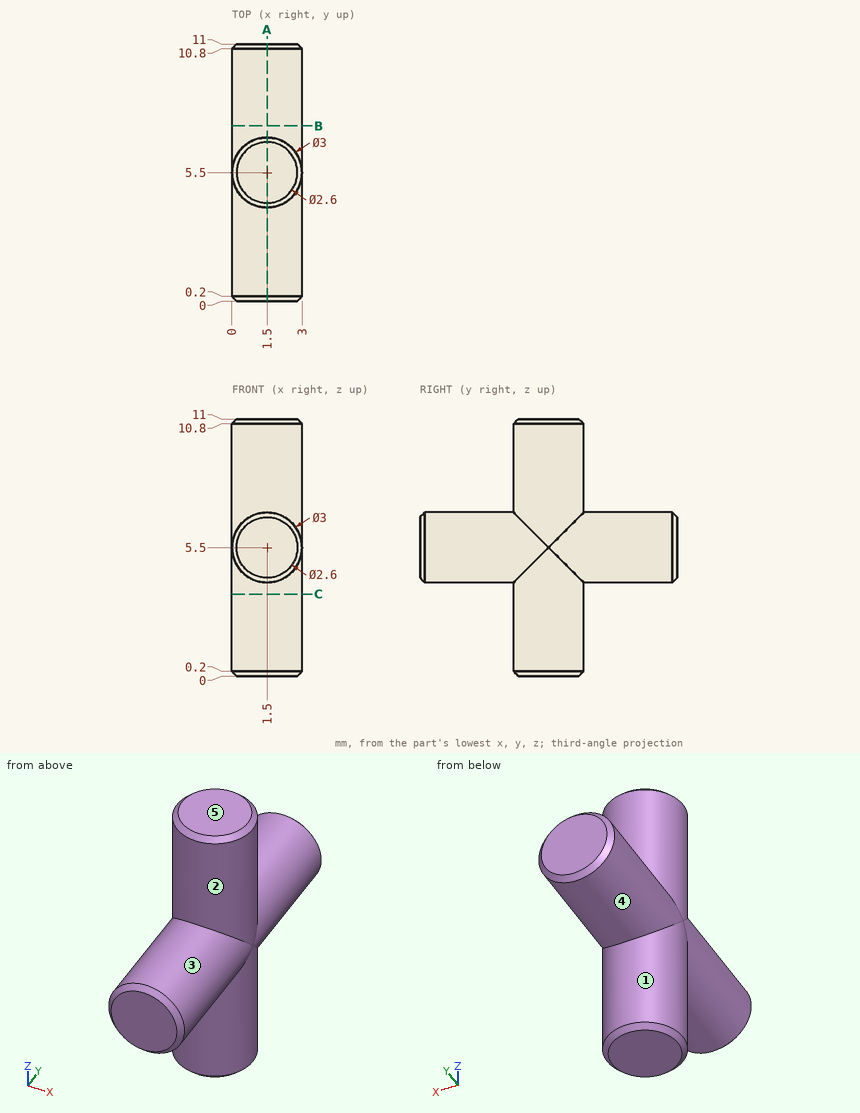
Job drawing, mm, ordinate dimensions from the low corner. One solid piece. A direction names the side the tool comes from. Round coordinates to 2 decimals unless told otherwise and drop trailing zeros. Loops run counter-clockwise (first coordinate to the right, second up) from the corner with the lowest first, then second, coordinate; pieces in that order, holes last. Notation, with made-up numbers: M -28,-20 L -10,-20 A14 cw -10,7 Z; hole C 16.25,42 d5. An arc over 180 degrees is marked long. One line per question, with ' | ' between items. Start each with the question number.
Item 1: Wall check: line 1 (Y direction, x = 1.4, z = 9.75); line 2 (X direction, y = 6.25, z = 7.5). Give the ranges that are in metal, low to high.
Item 2: Pin check, flat tip, straight feed: pin 1 Ø1 at (x, z) = (1.5, 9.5) entering from +Y. Stop position of the tip, or through.
Item 3: Which spindle directions (+Z, -Z, +X, -X, +Y, -Y) get a long thin tool onto all of the face, cutting with end or side? Do the marked faces 1, 2, 3, 4 and 5. Say none if no direction does.
Item 4: Cut at A-A, the plane x = 1.5. Write the cut outline in (y, z).
Item 5: Cut at B-B, the plane y = 7.5. Write the cut outline in (x, z).
Responses:
1) line 1: y = 4 to 7 | line 2: x = 0.2 to 2.8
2) pin 1: stops at y = 7
3) face 1: -Z | face 2: +Z | face 3: -Y | face 4: +Y | face 5: +Z, +X, -X, +Y, -Y
4) outline: M 0,4.2 L 0.2,4 L 4,4 L 4,0.2 L 4.2,0 L 6.8,0 L 7,0.2 L 7,4 L 10.8,4 L 11,4.2 L 11,6.8 L 10.8,7 L 7,7 L 7,10.8 L 6.8,11 L 4.2,11 L 4,10.8 L 4,7 L 0.2,7 L 0,6.8 Z
5) outline: C 1.5,5.5 d3
